Input: part model. Units: mm. Frame: model coordinates. Face numbers are marked on the shaded views. A direction names the side the tool comes from. Coordinates: 2 decimals unless noted, no trailing zeros. Loops run counter-clockwise (first coordinate to the right, second up) from the corner with the lowest first, then second, coordinate; pieces in that order, holes last. Notation, with made-up numbers: (78, 68.5) -> (93, 68.5) arc R22 cw to (93, 87.5) -> close; hole circle Ø5 at (18.5, -3). An arc over 180 degrees is marked (long way). Put each result on its own line as item: value. Start each with the question number.
1) Cut plane B-B (y = 29). Return the cut outline in (x, z).
2) Cut plane A-A (x = -29). Return the cut outline in (y, z), plus the area to 3 significant figures.
3) Material intervals for L1, parallel to X at y = 15, z = 2.75; L2, parallel to Z at x = -46.65, y = -2.5; L3, parallel to Y at x = 11.5, z = 4.75, sorted ascending.
4) Set-up query: the marked faces 1, 2 and 3. Return all of +Z, -Z, +X, -X, +Y, -Y with unobstructed straight access to the full face (end or side cutting, diameter ignored); none if empty.
5) Contact query for flat-ended pins moving along their axis: P1, Ø3, axis at x = -5.5, z = 2, coming from the -Y side; P2, Ø4, axis at x = -12.5, y = 23, coming from the -Z side; P3, Ø3, axis at y = -2.5, z = 3, coming from the -X side. Output: stop coordinate, or through.
from build123d import *

# Parameters (mm, degrees)
EXTRUDE_1_DEPTH     = 6
SKETCH_2_R          = 3.905124838
SKETCH_2_R_2        = 2.65
EXTRUDE_6_DEPTH     = 6
SKETCH_3_R          = 3.972728699
EXTRUDE_7_DEPTH     = 5
CUT_EXTRUDE_START   = -0.8
SKETCH_4_R          = 2.6
CUT_EXTRUDE_1_DEPTH = 4.2
SKETCH_5_W          = 40
SKETCH_5_H          = 17.5
CUT_EXTRUDE_2_DEPTH = 10


with BuildPart() as part:
    # 草图1 → 凸台-拉伸1 (new body)
    with BuildSketch(Plane.XY):
        Polygon((0, 0), (50, 0), (50, 65), (-50, 65), (-50, 0), align=None)
    extrude(amount=EXTRUDE_1_DEPTH)

    # 草图2 → 凸台-拉伸6 (add)
    with BuildSketch(Plane.ZY.offset(50)):
        with Locations((3, -2.5)):
            Circle(SKETCH_2_R)
        with Locations((3, -2.5)):
            Circle(SKETCH_2_R_2, mode=Mode.SUBTRACT)
    extrude(amount=-EXTRUDE_6_DEPTH)

    # 草图3 → 凸台-拉伸7 (add)
    with BuildSketch(Plane(origin=(50, 0, 0), x_dir=(0, 0, -1), z_dir=(1, 0, 0))):
        with Locations((-3.014231345, -2.587852917)):
            Circle(SKETCH_3_R)
    extrude(amount=-EXTRUDE_7_DEPTH)

    # 草图4 → 切除-拉伸1 (cut)
    with BuildSketch(Plane.ZY.offset(-45).offset(CUT_EXTRUDE_START)):
        with Locations((3.014231345, -2.587852917)):
            Circle(SKETCH_4_R)
    extrude(amount=-CUT_EXTRUDE_1_DEPTH, mode=Mode.SUBTRACT)

    # 草图5 → 切除-拉伸2 (cut)
    with BuildSketch(Plane.XY.offset(6)):
        with Locations((-15, 8.75)):
            Rectangle(SKETCH_5_W, SKETCH_5_H)
    extrude(amount=-CUT_EXTRUDE_2_DEPTH, mode=Mode.SUBTRACT)


solid = part.part
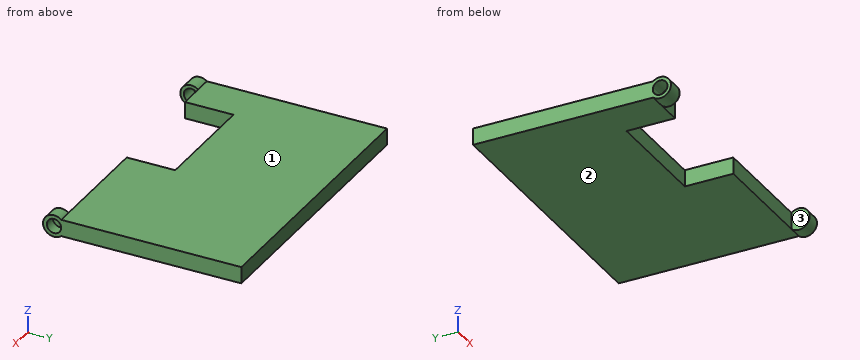
Results found:
1. outline: (-50, 0) -> (50, 0) -> (50, 6) -> (-50, 6) -> close
2. outline: (17.5, 0) -> (65, 0) -> (65, 6) -> (17.5, 6) -> close
2. area: 285 mm2
3. L1: x = -50 to -35, 5 to 50
3. L2: z = -0.91 to 0.35, 5.65 to 6.91
3. L3: y = 0 to 65
4. face 1: +Z, +X, -X, +Y
4. face 2: -Z, +X, -X, +Y
4. face 3: +Z, -Z, -Y
5. P1: stops at y = 17.5
5. P2: stops at z = 0
5. P3: stops at x = 45
